Can you work these out from the model? Positions are in its coordinate system, mm. Face numbers are marked on the shaded views. A direction names the side the tool comes from. Round coordinates to 2 decimals unless told otherwise and drop trailing zeros. Write each loop counter-clockwise with the first axis right and the second up, starting at its lowest first coordinate (ties: lowest second). Pieces come first, ordered by that corner, then holes. Notation, with made-up numbers: (-11.75, 24.5) - (23.25, 24.5) arc R12 ccw to (23.25, 44.5) - close; hole circle Ø4 at (61.25, -4). An arc over 180 degrees is marked (long way). One line per item, written item: value. Start each with the question number.
(1) On a 3-axis mill with a long thin cutter (end or side, diameter ignored), from which of +Z, -Z, +X, -X, +Y, -Y can I reach the whole of each face in a straight line? I mean the marked faces 3 and 4. Say none if no direction works.
(2) I want a section at C-C on y = -63. List the corners of the cut face in (x, z) for me, plus the area to 3 significant figures.
(3) I want a section at A-A on y = -11. List the corners of the cut face in (x, z) for me.
(4) If I drill on L1, parallel to X at y = -105, z = 1.75; L2, parallel to X at y = -8.5, z = -1.5; L3, parallel to Y at x = 23, z = 1, over which ranges is the centre line in solid material (lowest first)? Write a range as from..to.
(5) I'm going to push flat-ended pins straight in: pin 1 Ø1.8 at (x, y) = (11.5, -12.5) entering from -Z; pin 2 Ø1.8 at (x, z) = (1, -1.5) entering from +Y; pin 3 Ø5 at (x, y) = (-15, -10) entering from -Z. Where does each tip first touch, or does it pass through?
(6) Thinking about a two-plate mould opening in X: for the marked faces 1 and 2, which applies, +X half, -X half, draft (parallel to the pull), parting line (faces both ways), or undercut?
(7) I want a section at B-B on z = -1. List the corners of the cut face in (x, y) for me.
(8) I want a section at D-D on y = -36. List the corners of the cut face in (x, z) for me, plus the area to 3 significant figures.
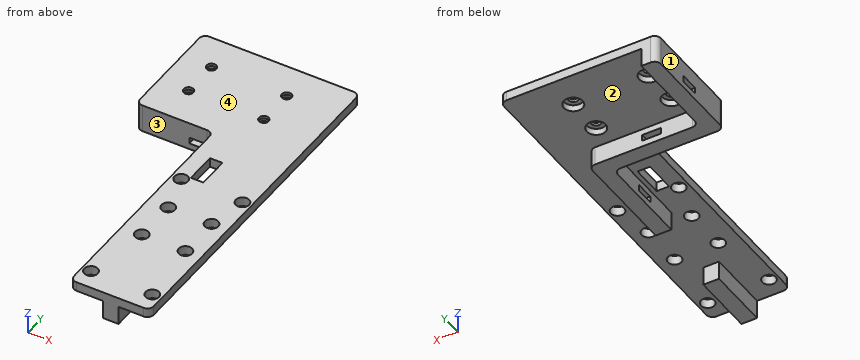
from build123d import *

# Parameters (mm, degrees)
BOSS_EXTRU_1_DEPTH                                 = 3
D_GAGEMENT_61_D                                    = 4.3053
CHAMBRAGE_POUR_VIS_T_TE_RONDE_BOMB_E_M_D           = 3.1
CHAMBRAGE_POUR_VIS_T_TE_RONDE_BOMB_E_M_CBORE_D     = 6
CHAMBRAGE_POUR_VIS_T_TE_RONDE_BOMB_E_M_CBORE_DEPTH = 2.1
ESQUISSE7_W                                        = 5
ESQUISSE7_H                                        = 20
BOSS_EXTRU_2_DEPTH                                 = 6
ENL_V_MAT_EXTRU_1_REACH                            = 117.582
ESQUISSE8_W                                        = 2
ESQUISSE8_H                                        = 6
ENL_V_MAT_EXTRU_2_REACH                            = 81.846
ESQUISSE9_W                                        = 6
ESQUISSE9_H                                        = 2
ENL_V_MAT_EXTRU_3_REACH                            = 122.972
ESQUISSE10_W                                       = 2
ESQUISSE10_H                                       = 6
CONG_1_R                                           = 2
D_GAGEMENT_65_D                                    = 4.3053
D_GAGEMENT_64_D                                    = 4.3053
ESQUISSE15_W                                       = 4
ESQUISSE15_H                                       = 10
ENL_V_MAT_EXTRU_4_DEPTH                            = 10


with BuildPart() as part:
    # Esquisse1 → Boss.-Extru.1 (new body)
    with BuildSketch(Plane.XY):
        Polygon((0, 0), (26.750817424, 0), (26.750817424, -109.991705561), (1.350817424, -109.991705561), (1.350817424, -35), (-23.249182576, -35), (-23.249182576, 0), align=None)
    extrude(amount=BOSS_EXTRU_1_DEPTH)

    # Dégagement #61 (through all)
    with Locations(Plane.XY.offset(3)):
        with Locations((21.588869509, -69.191705561), (7.788869509, -69.191705561), (7.729743851, -82.991705561), (21.650817424, -82.991705561)):
            Hole(D_GAGEMENT_61_D / 2)

    # Chambrage pour vis à tête ronde bombée M2.51 (through all)
    with Locations(Plane(origin=(0, 0, 0), x_dir=(-1, 0, 0), z_dir=(0, 0, -1))):
        with Locations((13.849182576, -23), (13.849182576, -11), (-10.150817424, -11), (-10.150817424, -23)):
            CounterBoreHole(CHAMBRAGE_POUR_VIS_T_TE_RONDE_BOMB_E_M_D / 2, CHAMBRAGE_POUR_VIS_T_TE_RONDE_BOMB_E_M_CBORE_D / 2, CHAMBRAGE_POUR_VIS_T_TE_RONDE_BOMB_E_M_CBORE_DEPTH)

    # Esquisse7 → Boss.-Extru.2 (add)
    with BuildSketch(Plane(origin=(0, 0, 0), x_dir=(-1, 0, 0), z_dir=(0, 0, -1))):
        Polygon((-11.750817424, -65), (-11.750817424, -35), (23.249182576, -35), (23.249182576, 0), (18.249182576, 0), (18.249182576, -30), (-16.750817424, -30), (-16.750817424, -65), align=None)
        with Locations((-14.250817424, -99.991705561)):
            Rectangle(ESQUISSE7_W, ESQUISSE7_H)
    extrude(amount=BOSS_EXTRU_2_DEPTH)

    # Esquisse8 → Enlèv. mat.-Extru.1 (cut, up to next)
    with BuildSketch(Plane.ZY.offset(-11.750817424), mode=Mode.PRIVATE) as enl_v_mat_extru_1_sk1:
        with Locations((-3, -51)):
            Rectangle(ESQUISSE8_W, ESQUISSE8_H)
    enl_v_mat_extru_1_tool1 = extrude(enl_v_mat_extru_1_sk1.sketch, amount=-ENL_V_MAT_EXTRU_1_REACH, mode=Mode.PRIVATE) & part.part
    add(enl_v_mat_extru_1_tool1.solids().sort_by_distance((11.750817, -51, -3))[0], mode=Mode.SUBTRACT)

    # Esquisse9 → Enlèv. mat.-Extru.2 (cut, up to next)
    with BuildSketch(Plane.XZ.offset(35), mode=Mode.PRIVATE) as enl_v_mat_extru_2_sk1:
        with Locations((-3.249182576, -3)):
            Rectangle(ESQUISSE9_W, ESQUISSE9_H)
    enl_v_mat_extru_2_tool1 = extrude(enl_v_mat_extru_2_sk1.sketch, amount=-ENL_V_MAT_EXTRU_2_REACH, mode=Mode.PRIVATE) & part.part
    add(enl_v_mat_extru_2_tool1.solids().sort_by_distance((-3.249183, -35, -3))[0], mode=Mode.SUBTRACT)

    # Esquisse10 → Enlèv. mat.-Extru.3 (cut, up to next)
    with BuildSketch(Plane.ZY.offset(23.249182576), mode=Mode.PRIVATE) as enl_v_mat_extru_3_sk1:
        with Locations((-3, -17)):
            Rectangle(ESQUISSE10_W, ESQUISSE10_H)
    enl_v_mat_extru_3_tool1 = extrude(enl_v_mat_extru_3_sk1.sketch, amount=-ENL_V_MAT_EXTRU_3_REACH, mode=Mode.PRIVATE) & part.part
    add(enl_v_mat_extru_3_tool1.solids().sort_by_distance((-23.249183, -17, -3))[0], mode=Mode.SUBTRACT)

    # Congé1
    cong_1_edges = [part.edges().sort_by_distance(p)[0] for p in [
        (26.750817424, 0, 1.5),
        (26.750817424, -109.991705561, 1.5),
        (1.350817424, -109.991705561, 1.5),
        (1.350817424, -35, 1.5),
        (-23.249182576, -35, -1.5),
        (-23.249182576, 0, -1.5),
        (-18.249182576, -30, -3),
        (16.750817424, -30, -3),
        (11.750817424, -35, -3),
    ]]
    fillet(cong_1_edges, radius=CONG_1_R)

    # Dégagement #65 (through all)
    with Locations(Plane(origin=(0, 0, 0), x_dir=(-1, 0, 0), z_dir=(0, 0, -1))):
        with Locations((-23.750817424, -103.791705561), (-4.190817424, -103.791705561)):
            Hole(D_GAGEMENT_65_D / 2)

    # Dégagement #64 (through all)
    with Locations(Plane(origin=(0, 0, 0), x_dir=(-1, 0, 0), z_dir=(0, 0, -1))):
        with Locations((-23.910817424, -56.791705561), (-4.350817424, -56.791705561)):
            Hole(D_GAGEMENT_64_D / 2)

    # Esquisse15 → Enlèv. mat.-Extru.4 (cut)
    with BuildSketch(Plane.XY.offset(3)):
        with Locations((8.350817424, -50)):
            Rectangle(ESQUISSE15_W, ESQUISSE15_H)
    extrude(amount=-ENL_V_MAT_EXTRU_4_DEPTH, mode=Mode.SUBTRACT)


solid = part.part
Established:
1. face 3: -Z, -X, -Y
1. face 4: +Z, +X, -X, +Y, -Y
2. outline: (1.35, 0) - (11.75, 0) - (11.75, -6) - (16.75, -6) - (16.75, 0) - (26.75, 0) - (26.75, 3) - (1.35, 3) - close
2. area: 106 mm2
3. outline: (-23.25, -6) - (-18.25, -6) - (-18.25, 0) - (-16.85, 0) - (-16.85, 2.1) - (-15.4, 2.1) - (-15.4, 3) - (-23.25, 3) - close; (-12.3, 2.1) - (-10.85, 2.1) - (-10.85, 0) - (7.15, 0) - (7.15, 2.1) - (8.6, 2.1) - (8.6, 3) - (-12.3, 3) - close; (11.7, 2.1) - (13.15, 2.1) - (13.15, 0) - (26.75, 0) - (26.75, 3) - (11.7, 3) - close
4. L1: 1.35..2.41, 5.97..21.97, 25.53..26.75
4. L2: -23.25..-18.25
4. L3: -109.99..-105.81, -101.77..-84.67, -81.31..-70.82, -67.57..-58.74, -54.84..0
5. pin 1: z = 2.1
5. pin 2: y = -30
5. pin 3: z = 0
6. face 1: -X half
6. face 2: draft
7. outline: (-23.25, -33) arc R2 ccw to (-21.25, -35) - (9.75, -35) arc R2 cw to (11.75, -37) - (11.75, -65) - (16.75, -65) - (16.75, -32) arc R2 ccw to (14.75, -30) - (-16.25, -30) arc R2 cw to (-18.25, -28) - (-18.25, 0) - (-21.25, 0) arc R2 ccw to (-23.25, -2) - close; (11.75, -109.99) - (16.75, -109.99) - (16.75, -89.99) - (11.75, -89.99) - close
8. outline: (1.08, 0) - (11.48, 0) - (11.48, -6) - (16.75, -6) - (16.75, 0) - (26.75, 0) - (26.75, 3) - (1.08, 3) - close
8. area: 109 mm2
